from build123d import *

# Parameters (mm, degrees)
F1_DEPTH = 2.5
F2_DEPTH = 2.5
F3_DEPTH = 0.5
F4_R     = 10


# Not quite as in the source:
# - a feature names something its author has since deleted; it is built from what else it names


with BuildPart() as f1:
    # F0 (on Top) → F1 (new body, symmetric)
    with BuildSketch(Plane.XY):
        with BuildLine():
            Line((-41.7, 5.2), (-3.6, 5.2))
            Line((-3.6, 5.2), (-3.6, 5.5))
            ThreePointArc((-3.6, 5.5), (-7.2954363748, 6.8447474533), (-9.2623758265, 10.25))
            Line((-9.2623758265, 10.25), (-19.5376241735, 10.25))
            ThreePointArc((-19.5376241735, 10.25), (-30.9280520686, 11.7519158285), (-19.45, 11.25))
            Line((-19.45, 11.25), (-9.35, 11.25))
            ThreePointArc((-9.35, 11.25), (-3.6, 17), (2.15, 11.25))
            Line((2.15, 11.25), (7.2, 11.25))
            Line((7.2, 11.25), (12.25, 11.25))
            ThreePointArc((12.25, 11.25), (18, 17), (23.75, 11.25))
            ThreePointArc((23.75, 11.25), (18.5019158285, 5.5219479314), (12.3376241735, 10.25))
            Line((12.3376241735, 10.25), (7.2, 10.25))
            Line((7.2, 10.25), (7.2, 5.2))
            Line((7.2, 5.2), (56.1, 5.2))
            Line((56.1, 5.2), (56.1, 22.3))
            Line((56.1, 22.3), (-41.7, 22.3))
            Line((-41.7, 22.3), (-41.7, 5.2))
        make_face()
        with BuildLine():
            ThreePointArc((45.35, 11.25), (39.6, 5.5), (33.85, 11.25))
            ThreePointArc((33.85, 11.25), (39.6, 17), (45.35, 11.25))
        make_face(mode=Mode.SUBTRACT)
        with BuildLine():
            Line((-3.6, 5.5), (-3.6, 5.2))
            Line((-3.6, 5.2), (7.2, 5.2))
            Line((7.2, 5.2), (7.2, 10.25))
            Line((7.2, 10.25), (2.0623758265, 10.25))
            ThreePointArc((2.0623758265, 10.25), (0.0954363748, 6.8447474533), (-3.6, 5.5))
        make_face()
        with BuildLine():
            Line((-19.5376241735, 10.25), (-9.2623758265, 10.25))
            ThreePointArc((-9.2623758265, 10.25), (-9.3280520686, 10.7480841715), (-9.35, 11.25))
            Line((-9.35, 11.25), (-19.45, 11.25))
            ThreePointArc((-19.45, 11.25), (-19.4719479314, 10.7480841715), (-19.5376241735, 10.25))
        make_face()
        with BuildLine():
            ThreePointArc((2.15, 11.25), (2.1280520686, 10.7480841715), (2.0623758265, 10.25))
            Line((2.0623758265, 10.25), (7.2, 10.25))
            Line((7.2, 10.25), (7.2, 11.25))
            Line((7.2, 11.25), (2.15, 11.25))
        make_face()
        with BuildLine():
            Line((7.2, 11.25), (7.2, 10.25))
            Line((7.2, 10.25), (12.3376241735, 10.25))
            ThreePointArc((12.3376241735, 10.25), (12.2719479314, 10.7480841715), (12.25, 11.25))
            Line((12.25, 11.25), (7.2, 11.25))
        make_face()
    extrude(amount=F1_DEPTH, both=True)



with BuildPart() as f1b:
    # F0 (on Top) → F1, piece 2 (new body, symmetric)
    with BuildSketch(Plane.XY):
        Polygon((56.1, -5.2), (-3.6, -5.2), (-41.7, -5.2), (-41.7, -22.3), (56.1, -22.3), align=None)
        with BuildLine():
            ThreePointArc((-9.2623758265, -10.25), (-7.2954363748, -6.8447474533), (-3.6, -5.5))
            ThreePointArc((-3.6, -5.5), (0.0954363748, -6.8447474533), (2.0623758265, -10.25))
            Line((2.0623758265, -10.25), (12.3376241735, -10.25))
            ThreePointArc((12.3376241735, -10.25), (18.5019158285, -5.5219479314), (23.75, -11.25))
            ThreePointArc((23.75, -11.25), (18, -17), (12.25, -11.25))
            Line((12.25, -11.25), (2.15, -11.25))
            ThreePointArc((2.15, -11.25), (-3.6, -17), (-9.35, -11.25))
            Line((-9.35, -11.25), (-19.45, -11.25))
            ThreePointArc((-19.45, -11.25), (-30.9280520686, -11.7519158285), (-19.5376241735, -10.25))
            Line((-19.5376241735, -10.25), (-9.2623758265, -10.25))
        make_face(mode=Mode.SUBTRACT)
        with BuildLine():
            ThreePointArc((45.35, -11.25), (39.6, -17), (33.85, -11.25))
            ThreePointArc((33.85, -11.25), (39.6, -5.5), (45.35, -11.25))
        make_face(mode=Mode.SUBTRACT)
        with BuildLine():
            Line((12.3376241735, -10.25), (2.0623758265, -10.25))
            ThreePointArc((2.0623758265, -10.25), (2.1280520686, -10.7480841715), (2.15, -11.25))
            Line((2.15, -11.25), (12.25, -11.25))
            ThreePointArc((12.25, -11.25), (12.2719479314, -10.7480841715), (12.3376241735, -10.25))
        make_face()
        with BuildLine():
            ThreePointArc((-9.35, -11.25), (-9.3280520686, -10.7480841715), (-9.2623758265, -10.25))
            Line((-9.2623758265, -10.25), (-19.5376241735, -10.25))
            ThreePointArc((-19.5376241735, -10.25), (-19.4719479314, -10.7480841715), (-19.45, -11.25))
            Line((-19.45, -11.25), (-9.35, -11.25))
        make_face()
    extrude(amount=F1_DEPTH, both=True)


with BuildPart() as f1_1:
    add(f1.part)

    add(f1b.part)  # F2 merges F1b
    # F0 (on Top) → F2 (join)
    with BuildSketch(Plane.XY):
        Polygon((-3.6, -5.2), (-3.6, 0), (-3.6, 5.2), (-41.7, 5.2), (-41.7, -5.2), align=None)
        Polygon((-3.6, 5.2), (-3.6, 0), (-3.6, -5.2), (56.1, -5.2), (56.1, 0), (56.1, 5.2), (7.2, 5.2), align=None)
    extrude(amount=F2_DEPTH)

    # F0 (on Top) → F3 (join)
    with BuildSketch(Plane.XY):
        Polygon((-3.6, 5.2), (-3.6, 0), (-3.6, -5.2), (56.1, -5.2), (56.1, 0), (56.1, 5.2), (7.2, 5.2), align=None)
        Polygon((-3.6, -5.2), (-3.6, 0), (-3.6, 5.2), (-41.7, 5.2), (-41.7, -5.2), align=None)
    extrude(amount=-F3_DEPTH)

    # F4
    f4_edges = [f1_1.edges().sort_by_distance(p)[0] for p in [
        (56.1, -22.3, 0),
        (-41.7, -22.3, 0),
        (-41.7, 22.3, 0),
        (56.1, 22.3, 0),
    ]]
    fillet(f4_edges, radius=F4_R)


solid = f1_1.part
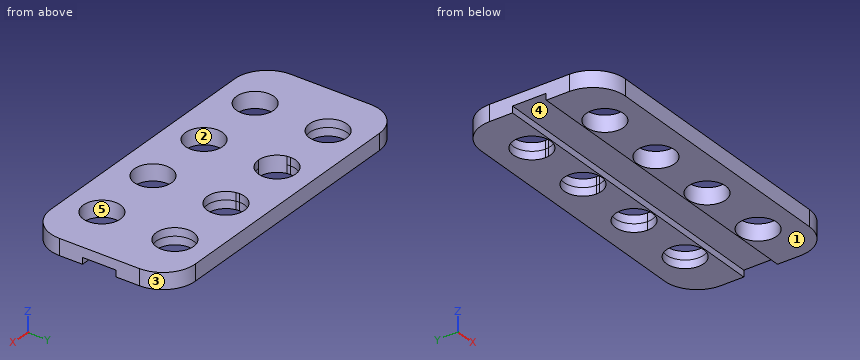
Build history of the part. All positions in model axes, mm. Face numbers are marked on the shaded views. A direction names the side the tool comes from. Round coordinates to 2 decimals unless told otherwise and drop trailing zeros. Loops run counter-clockwise (first coordinate to the right, second up) from the corner with the lowest first, then second, coordinate; pieces in that order, holes last. Notation, with made-up numbers: (75.25, -17) -> (91.25, -17) arc R14 cw to (91.25, -7) -> close; hole circle Ø2 at (62, 4.25). An arc over 180 degrees is marked (long way). One line per item, written item: value. Start each with the question number.
Q1. Two-plate mould, pull along X, no slides. Class the marked faces 1, 2 and 3: released by +X, released by -X, zero draft, split by the parting line, or undercut.
Q2. Drop flat-ended pins along their axis: pin 1 Ø10.5 at (x, y) = (39.6, -11.25) entering from -Z; pin 2 Ø5 at (x, y) = (11, 2) entering from -Z. Give the stop position or say it passes through.
Q3. Cut at A-A on x = 39.6. List the corners of the cut face in (y, z).
Q4. 3-axis set-ups, long thin cutter, end or side, ignore diameter. For the marked faces 4 and 5: which of +Z, -Z, +X, -X, +Y, -Y reach the whole face in a straight line?
Q5. Cut at C-C on y = -11.25. List the corners of the cut face in (x, z).
Q6. Cut at D-D on y = 16. List the corners of the cut face in (x, z).
Q7. Cut at B-B on z = 0.95. Count the separate pieces of the cut face and the enclosed holes in it, plus the area to 3 significant figures.
Q8. Probe line 1 along Y through (x, z) = (6, -1.5); line 2 along Y through (x, z) = (39.6, -1); line 3 along X through (y, z) = (6, 0.2). List the from-to ranges inside material, lowest first.
Computed:
1. face 1: zero draft
1. face 2: undercut
1. face 3: released by +X
2. pin 1: through
2. pin 2: z = -0.5
3. outline: (-22.3, -2.5) -> (-17, -2.5) -> (-17, 2.5) -> (-22.3, 2.5) -> close; (-5.5, -2.5) -> (-5.2, -2.5) -> (-5.2, -0.5) -> (5.2, -0.5) -> (5.2, -2.5) -> (5.5, -2.5) -> (5.5, 2.5) -> (-5.5, 2.5) -> close; (17, -2.5) -> (22.3, -2.5) -> (22.3, 2.5) -> (17, 2.5) -> close
4. face 4: -Z, +X, -X
4. face 5: +Z, -Z
5. outline: (-41.7, -2.5) -> (-30.95, -2.5) -> (-30.95, 2.5) -> (-41.7, 2.5) -> close; (-19.45, -2.5) -> (-9.35, -2.5) -> (-9.35, 2.5) -> (-19.45, 2.5) -> close; (2.15, -2.5) -> (12.25, -2.5) -> (12.25, 2.5) -> (2.15, 2.5) -> close; (23.75, -2.5) -> (33.85, -2.5) -> (33.85, 2.5) -> (23.75, 2.5) -> close; (45.35, -2.5) -> (56.1, -2.5) -> (56.1, 2.5) -> (45.35, 2.5) -> close
6. outline: (-40.99, -2.5) -> (-28.44, -2.5) -> (-28.44, 2.5) -> (-40.99, 2.5) -> close; (-21.96, -2.5) -> (-6.84, -2.5) -> (-6.84, 2.5) -> (-21.96, 2.5) -> close; (-0.36, -2.5) -> (14.76, -2.5) -> (14.76, 2.5) -> (-0.36, 2.5) -> close; (21.24, -2.5) -> (36.36, -2.5) -> (36.36, 2.5) -> (21.24, 2.5) -> close; (42.84, -2.5) -> (55.39, -2.5) -> (55.39, 2.5) -> (42.84, 2.5) -> close
7. separate pieces: 1
7. enclosed holes: 8
7. area: 3,450 mm²
8. line 1: -22.3 to -5.2, 5.2 to 22.3
8. line 2: -22.3 to -17, -5.5 to -5.2, 5.2 to 5.5, 17 to 22.3
8. line 3: -41.7 to -27.55, -22.85 to -5.95, -1.25 to 15.65, 20.35 to 37.25, 41.95 to 56.1
